Part model, mm, in its own coordinate system. A direction names the side the tool comes from. Give positions to 0.01 mm unless a question says otherwise; leave off trailing zeros. Order: outer loops, then holes, each group sorted by start corner. A loop starts at its lowest first (then second) coordinate and runs counter-clockwise, first axis right, second up. Notation, with made-up numbers: (54.5, 53) - (104.5, 53) arc R19 ccw to (104.5, 73) - close; hole circle Ø11 at (83.25, 19). An arc over 180 degrees is marked (long way). One line per item, written item: value.
```python
from build123d import *

# Parameters (mm, degrees)
SKETCH_1_W          = 75
SKETCH_1_H          = 100
EXTRUDE_1_DEPTH     = 6
SKETCH_3_R          = 0.75
CUT_EXTRUDE_1_DEPTH = 7
SKETCH_4_W          = 12.62553929
SKETCH_4_H          = 13.5
SKETCH_4_W_2        = 12.874809427
SKETCH_4_W_3        = 12.837463025
CUT_EXTRUDE_2_DEPTH = 75.027022093


with BuildPart() as part:
    # Эскиз1 → Вытянуть1 (new body)
    with BuildSketch(Plane(origin=(0, 0, 0), x_dir=(1, 0, 0), z_dir=(0, 1, 0))):
        with Locations((2.5, 12)):
            Rectangle(SKETCH_1_W, SKETCH_1_H)
    extrude(amount=EXTRUDE_1_DEPTH)

    # Эскиз3 → Вырез-Вытянуть1 (cut)
    with BuildSketch(Plane(origin=(40, 0, 0), x_dir=(0, 0, -1), z_dir=(1, 0, 0))):
        with Locations((-28.708129091, 3)):
            Circle(SKETCH_3_R)
    extrude(amount=-CUT_EXTRUDE_1_DEPTH, mode=Mode.SUBTRACT)

    # Эскиз4 → Вырез-Вытянуть2 (cut, through all)
    with BuildSketch(Plane.XZ):
        with Locations((43.312769645, 26.25)):
            Rectangle(SKETCH_4_W, SKETCH_4_H)
        with Locations((43.437404714, -50.25)):
            Rectangle(SKETCH_4_W_2, SKETCH_4_H)
        Polygon((-35, -38), (-35, -62), (-25, -62), (-25, -58), (-22, -58), (-22, -44.5), (-25, -44.5), (-25, -38), align=None)
        with Locations((43.418731513, 0.75)):
            Rectangle(SKETCH_4_W_3, SKETCH_4_H)
        with Locations((43.418731513, -24.75)):
            Rectangle(SKETCH_4_W_3, SKETCH_4_H)
        Polygon((-35, 14), (-25, 14), (-25, 20.5), (-22, 20.5), (-22, 34), (-25, 34), (-25, 38), (-35, 38), align=None)
    extrude(amount=-CUT_EXTRUDE_2_DEPTH, mode=Mode.SUBTRACT)


solid = part.part
```
1) Pin check, flat tips, straight feed: pin 1 (2 mm diameter, centred on y = 3, z = 28.71, fed in from -X); pin 2 (3 mm diameter, centred on y = 2.5, z = 36.5, fed in from -X); pin 3 (1 mm diameter, centred on y = 2, z = -28.5, fed in from +X). Stop position of each tip, or through.
Outcome:
pin 1: stops at x = -22
pin 2: stops at x = -25
pin 3: stops at x = 37
2) Cut at C-C, the plane z = 4.5. Give the cut face in (x, y).
Outcome:
outline: (-35, 0) - (37, 0) - (37, 6) - (-35, 6) - close
3) Which spindle directions (+Z, -Z, +X, -X, +Y, -Y) get a long thin tool onto all of the face, cutting with end or side? Do faces 4 (the flat face through (-25, 3, 36)), 5 (the flat face through (-23, 3, 34)), 6 (the flat face through (-30, 3, -38)), 7 (the flat face through (38, 3, 19.5)), 8 (the flat face through (40, 3, -12)). Say none if no direction does.
Outcome:
face 4: +Z, -X, +Y, -Y
face 5: -X, +Y, -Y
face 6: -Z, -X, +Y, -Y
face 7: +X, +Y, -Y
face 8: +Z, -Z, +X, +Y, -Y
4) Cut at B-B, the plane x = -27.5. Give the cut face in (y, z), then the cut area to 3 significant figures.
Outcome:
outline: (0, -38) - (6, -38) - (6, 14) - (0, 14) - close
area: 312 mm^2
5) Drill centre lines: line 1 along Z through (x, y) = (-23.5, 2.9); line 2 along X through (y, z) = (4.9, 25); line 3 along X through (y, z) = (1.25, -40.5). Where is each one in solid material? Low to high. Write a range as from..to.
Outcome:
line 1: z = -62..-58, -44.5..20.5, 34..38
line 2: x = -22..37
line 3: x = -25..40
6) Mould opens along Z. For faces 1 (the flat face through (38, 3, 33)), 2 (the flat face through (7, 3, -62)), 3 (the flat face through (-25, 3, 17)) say: released by +Z, released by -Z, zero draft, split by the parting line, or undercut.
Outcome:
face 1: undercut
face 2: released by -Z
face 3: zero draft
